from build123d import *

# Parameters (mm, degrees)
ESBO_O1_W                  = 34.6
ESBO_O1_H                  = 26
RESSALTO_EXTRUS_O1_DEPTH   = 7
ESBO_O10_W                 = 34.6
ESBO_O10_H                 = 2.5
RESSALTO_EXTRUS_O4_DEPTH   = 7
CHANFRO1_SIZE              = 7
CHANFRO2_SIZE2             = 7
CHANFRO2_SIZE              = 2.54779164
ESBO_O12_R                 = 1.65
RESSALTO_EXTRUS_O5_DEPTH   = 30
RESSALTO_EXTRUS_O6_START   = 3
RESSALTO_EXTRUS_O6_DEPTH   = 8
CORTE_EXTRUS_O2_DEPTH      = 40.089640571
CORTE_EXTRUS_O2_DEPTH_BACK = 40.089640571
CHANFRO3_SIZE              = 9
CHANFRO3_SIZE_2            = 19.300562285
CORTE_EXTRUS_O3_START      = -24
ESBO_O17_R                 = 4.5
CORTE_EXTRUS_O3_DEPTH      = 18


# Some blends are built 0.0001 mm under size
with BuildPart() as part:
    # Esboço1 → Ressalto-extrusão1 (new body)
    with BuildSketch(Plane.XY):
        Rectangle(ESBO_O1_W, ESBO_O1_H)
    extrude(amount=RESSALTO_EXTRUS_O1_DEPTH)

    # Esboço10 → Ressalto-extrusão4 (add)
    with BuildSketch(Plane(origin=(0, 0, 0), x_dir=(-1, 0, 0), z_dir=(0, 0, -1))):
        Polygon((-17.3, -19.5), (0, -26.5), (17.3, -19.5), (17.3, -13), (-17.3, -13), align=None)
        with Locations((0, 14.25)):
            Rectangle(ESBO_O10_W, ESBO_O10_H)
    extrude(amount=-RESSALTO_EXTRUS_O4_DEPTH)

    # Chanfro1
    chanfro1_edges = [part.edges().sort_by_distance(p)[0] for p in [
        (8.65, -23, 7),
        (-8.65, -23, 7),
    ]]
    chamfer(chanfro1_edges, length=CHANFRO1_SIZE - 0.0001)  # a hair under: the kernel refuses the full size

    # Chanfro2
    chanfro2_edges = [part.edges().sort_by_distance(p)[0] for p in [
        (0, 15.5, 7),
    ]]
    chanfro2_side = [part.faces().sort_by_distance(p)[0] for p in [
        (0, 15.449044167, 7),
    ]]
    chamfer(chanfro2_edges, length=CHANFRO2_SIZE - 0.0001, length2=CHANFRO2_SIZE2 - 0.0001, reference=chanfro2_side[0])  # a hair under: the kernel refuses the full size

    # Esboço12 → Ressalto-extrusão5 (add)
    # profile 1 of 2: a face of its own
    with BuildSketch(Plane(origin=(0, 0, 0), x_dir=(1, 0, 0), z_dir=(0, 1, 0))):
        with BuildLine():
            Line((-17, -19), (-17, -7))
            Line((-17, -7), (-8, -7))
            Line((-8, -7), (-8, -19))
            ThreePointArc((-8, -19), (-12.5, -23.5), (-17, -19))
        make_face()
        with Locations(Location((-12.5, -19, 0), (0, 0, 270))):
            Circle(ESBO_O12_R, mode=Mode.SUBTRACT)
    # profile 2 of 2: a face of its own
    with BuildSketch(Plane(origin=(0, 0, 0), x_dir=(1, 0, 0), z_dir=(0, 1, 0))):
        with BuildLine():
            Line((8, -7), (8, -19))
            ThreePointArc((8, -19), (12.5, -23.5), (17, -19))
            Line((17, -19), (17, -7))
            Line((17, -7), (8, -7))
        make_face()
        with Locations(Location((12.5, -19, 0), (0, 0, 90))):
            Circle(ESBO_O12_R, mode=Mode.SUBTRACT)
    extrude(amount=RESSALTO_EXTRUS_O5_DEPTH)

    # Esboço15 → Ressalto-extrusão6 (add)
    with BuildSketch(Plane(origin=(0, 0, 0), x_dir=(1, 0, 0), z_dir=(0, 1, 0)).offset(RESSALTO_EXTRUS_O6_START)):
        Polygon((-22, -11.5), (-22, -8.5), (-17, -8.5), (-17, -7), (-8, -7), (-8, -11.5), align=None)
        Polygon((17, -8.5), (17, -7), (8, -7), (8, -11.5), (22, -11.5), (22, -8.5), align=None)
    extrude(amount=RESSALTO_EXTRUS_O6_DEPTH)

    # Esboço16 → Corte-extrusão2 (cut, two sides: drawn at the far end of the back side and taken through both)
    with BuildSketch(Plane.XY.offset(11.5).offset(-CORTE_EXTRUS_O2_DEPTH_BACK)):
        Polygon((-17.3, 3), (-19.8, 5.5), (-19.8, 3), align=None)
        Polygon((19.8, 3), (17.3, 3), (19.8, 5.5), align=None)
    extrude(amount=CORTE_EXTRUS_O2_DEPTH + CORTE_EXTRUS_O2_DEPTH_BACK, mode=Mode.SUBTRACT)

    # Chanfro3
    # the kernel refuses this chamfer: 19.300562285, 9 mm, written as the material it takes off along each edge
    with BuildSketch(Plane(origin=(-67.007283464, 30, 7), x_dir=(0, 0.07481330637060048, 0.9971975577536772), z_dir=(1, 0, 0))) as chanfro3_piece_1_section:
        Polygon((CHANFRO3_SIZE * 0.997197557754, CHANFRO3_SIZE * 0.0748133063706), (-CHANFRO3_SIZE_2 * 0.074813306369, CHANFRO3_SIZE_2 * 0.997197557732), (0, 0), align=None)
    chanfro3_piece_1 = extrude(amount=109.014566928, mode=Mode.PRIVATE)
    chanfro3_piece_1 = split(chanfro3_piece_1, bisect_by=Plane(origin=(-12.5, 13.283132455, 6.091045576), z_dir=(0, 0.9396953649145792, 0.34201260380000037)), keep=Keep.TOP, mode=Mode.PRIVATE)
    add(chanfro3_piece_1, mode=Mode.SUBTRACT)
    with BuildSketch(Plane(origin=(67.007283464, 30, 7), x_dir=(0, -0.9998669641130703, -0.01631116413111024), z_dir=(-1, 0, 0))) as chanfro3_piece_2_section:
        Polygon((CHANFRO3_SIZE_2 * 0.999866964092, CHANFRO3_SIZE_2 * 0.0163111641308), (-CHANFRO3_SIZE * 0.0163111641311, CHANFRO3_SIZE * 0.999866964113), (0, 0), align=None)
    chanfro3_piece_2 = extrude(amount=109.014566928, mode=Mode.PRIVATE)
    chanfro3_piece_2 = split(chanfro3_piece_2, bisect_by=Plane(origin=(12.5, 13.283132455, 6.091045576), z_dir=(0, 0.9396953649145792, 0.34201260380000037)), keep=Keep.TOP, mode=Mode.PRIVATE)
    add(chanfro3_piece_2, mode=Mode.SUBTRACT)

    # Esboço17 → Corte-extrusão3 (cut)
    with BuildSketch(Plane.XZ.offset(CORTE_EXTRUS_O3_START)):
        with Locations((-12.5, 19)):
            Circle(ESBO_O17_R)
        with Locations((12.5, 19)):
            Circle(ESBO_O17_R)
    extrude(amount=CORTE_EXTRUS_O3_DEPTH, mode=Mode.SUBTRACT)


solid = part.part
Verification items for the finished model (mm, model axes). A direction names the side the tool comes from. Give positions to 0.01 mm unless a question says otherwise; leave off trailing zeros. Order: outer loops, then holes, each group sorted by start corner. A loop starts at its lowest first (then second) coordinate and runs counter-clockwise, first axis right, second up. Notation, with made-up numbers: M -6.5,29.25 L 0.5,29.25 A8 cw 0.5,36.25 Z; hole C 46,-33 d7. An arc over 180 degrees is marked long. Answer as a JSON object with one key per item and string values. Group by question number.
1) Mould release check, pull along Y, two halves, no side actions. Record for faces 5 (the face through (14.4, 6, 19.1)), 6 (the face through (12.4, 15.1, 14.5)), 7 (the face through (0, -3, 7)), 8 (the face through (-19, 11, 10)): released by +Y, released by -Y, zero draft, split by the parting line, or undercut.
2) Scan lines: line 1 along X through (y, z) = (27.4, 19); line 2 along Y through (x, z) = (13, 20.75); line 3 along Z through (x, y) = (-11.5, -4.5). Record each from-to range of solid material in increasing order. Write a range as [from, to].
3) Cross-section at A-A (z = 10.5). Enter the section's corners in (x, y).
4) Cross-section at B-B (x = 12.5). Give the number of separate pieces and of enclosed holes in the cut face, then the cut area to 3 significant figures.
5) Depth check by flat-ended pin: pin 1 Ø4.5 at (x, z) = (12.5, 19.5) entering from -Y; pin 2 Ø5.5 at (y, z) = (-6.5, 3) entering from -X; pin 3 Ø2.5 at (x, z) = (-19, 10.5) entering from +Y; pin 4 Ø6 at (x, y) = (10, 7.5) entering from -Z. Enter the tip coordinate at first touch or a pass-through.
6) Access from +Z, -Z, +X, -X, +Y, -Y to the whole of each face (thin tool, end or side, straight path). Record for faces 1 (the face through (-17.3, -2, 3)), 2 (the face through (-12.6, 15.1, 14.5)), 3 (the face through (12, 0, 15)), 4 (the face through (-19, 7, 11.5)).
7) Cross-section at D-D (y = -14.5). Enter the section's corners in (x, z).
8) Cross-section at C-C (y = 21). Enter the section's corners in (x, z).
Result sheet:
{
 "1": {"face 5": "undercut", "face 6": "undercut", "face 7": "zero draft", "face 8": "released by +Y"},
 "2": {"line 1": "x = [-17, -14.15], [-10.85, -8], [8, 10.85], [14.15, 17]", "line 2": "y = [0, 6], [24, 30]", "line 3": "z = [0, 7]"},
 "3": {"outline": "M -22,3 L -19.8,3 L -19.8,5.5 L -17.3,3 L -17,3 L -17,0 L -8,0 L -8,18.21 L -17,18.21 L -17,11 L -22,11 Z; M 8,0 L 17,0 L 17,3 L 17.3,3 L 19.8,5.5 L 19.8,3 L 22,3 L 22,11 L 17,11 L 17,18.21 L 8,18.21 Z"},
 "4": {"separate pieces": "3", "enclosed holes": "0", "area": "431 mm2"},
 "5": {"pin 1": "stops at y = 0", "pin 2": "stops at x = -17.3", "pin 3": "stops at y = 11", "pin 4": "stops at z = 0"},
 "6": {"face 1": "-Z, -X, +Y, -Y", "face 2": "+Z", "face 3": "+Z, +X, -X, -Y", "face 4": "+Z, -X, +Y, -Y"},
 "7": {"outline": "M -17.3,0 L 17.3,0 L 17.3,4.64 L 10.99,7 L -10.99,7 L -17.3,4.64 Z"},
 "8": {"outline": "M -17,11.8 L -8,11.8 L -8,19 A4.5 cw -17,19 Z; M 8,11.8 L 17,11.8 L 17,19 A4.5 cw 8,19 Z"}
}
